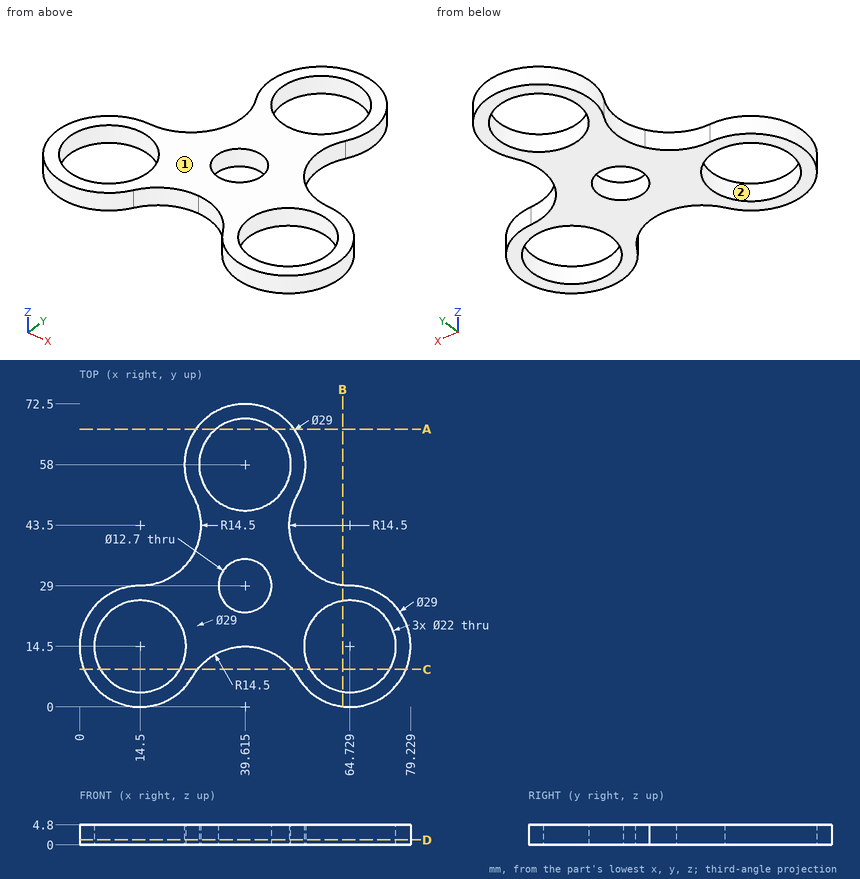
Design review of the part shown in the three views and the two pictorial views. Dimensions are in mm from the part's minimum x, y and z. Coordinates: 2 decimals unless noted, no trailing zeros. Order: outer loops, then holes, each group sorted by start corner. A loop starts at its lowest first (then second) coordinate and runs counter-clockwise, first axis right, second up.
1) Take a section at B-B, the plane x = 63. Give the boundary of the cut face in (y, z), and give its area (3 significant figures).
2) Mouldability with a two-part tool opening along X and no side actions: class the marked faces 1 and 2 as +X half, -X half, draft (parallel to the pull), parting line (faces both ways), or undercut.
3) Take a section at A-A, the plane y = 66.5. Give the boundary of the cut face in (x, z).
4) Clearance check with flat-ended pins moving along their axes: pin 1 (1.5 mm diameter, centred on x = 28, z = 2, fed in from -Y) (1 decimal); pin 2 (13 mm diameter, centred on x = 64.73, y = 14.5, fed in from -Z); pin 3 (2 mm diameter, centred on y = 11, z = 2, fed in from -X); pin 4 (1 mm diameter, centred on x = 45.5, z = 2.5, fed in from +Y). State where each tip first meets the part, or that it passes through.
5) Wall thickness on line 1 along Y through (x, z) = (34.5, 0.95) (1 decimal); line 2 along X through (y, z) = (58, 1.3) (1 decimal); line 3 along Y through (x, z) = (37, 1.5) (1 decimal): over which ranges is each line inside the solid? List them lowest first.
6) Take a section at D-D, the plane z = 1.25. State how many separate pieces and enclosed holes the cut face has, and give its area (3 significant figures).
7) Take a section at C-C, the plane y = 9. Give the boundary of the cut face in (x, z) (1 decimal).
Returned:
1. outline: (0.1, 0) - (3.64, 0) - (3.64, 4.8) - (0.1, 4.8) - close; (25.36, 0) - (29.1, 0) - (29.1, 4.8) - (25.36, 4.8) - close
1. area: 34.9 mm2
2. face 1: draft
2. face 2: undercut
3. outline: (27.87, 0) - (32.63, 0) - (32.63, 4.8) - (27.87, 4.8) - close; (46.6, 0) - (51.36, 0) - (51.36, 4.8) - (46.6, 4.8) - close
4. pin 1: stops at y = 7.6
4. pin 2: passes through
4. pin 3: stops at x = 0.22
4. pin 4: stops at y = 71.46
5. line 1: y = 13.6 to 25.2, 32.8 to 48.3, 67.7 to 71.6
5. line 2: x = 25.1 to 28.6, 50.6 to 54.1
5. line 3: y = 14.3 to 23.2, 34.8 to 47.3, 68.7 to 72.3
6. separate pieces: 1
6. enclosed holes: 4
6. area: 1,580 mm2
7. outline: (1.1, 0) - (5, 0) - (5, 4.8) - (1.1, 4.8) - close; (24, 0) - (28.2, 0) - (28.2, 4.8) - (24, 4.8) - close; (51, 0) - (55.2, 0) - (55.2, 4.8) - (51, 4.8) - close; (74.3, 0) - (78.1, 0) - (78.1, 4.8) - (74.3, 4.8) - close
